Verification items for the finished model (mm, model axes). Round coordinates to 2 decimals unless told otherwise and drop trailing zeros. Order: outer loops, then holes, each group sorted by start corner. A loop starts at its lowest first (then second) coordinate and runs counter-clockwise, first axis right, second up. Notation, with made-up numbers: M 46,17.25 L 53,17.25 A23 cw 53,42.25 Z; hole C 68,1.25 d1. An arc over 180 degrees is marked long. Use CSV: the item, a comma, the result in double quotes. Start each with the question number.
Q1. Sectioned sample at A-A (y = 61.5). Enter the section's corners in (x, z).
Q2. Scan lines: line 1 (X direction, y = 17.5, z = 0.9); line 2 (X direction, y = 81, z = 1.25); line 3 (Z direction, x = -1, y = 69). Record each from-to range of solid material in increasing order.
Q3. Sectioned sample at C-C (z = 3.8). Enter the section's corners in (x, y) (3 decimals), and give its area (3 significant figures).
Q4. Sectioned sample at B-B (x = -1.5). Enter the section's corners in (y, z).
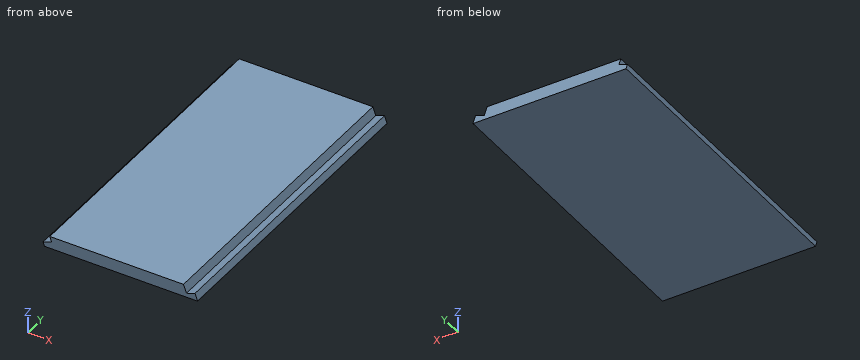
```python
from build123d import *

# Parameters (mm, degrees)
BOX018_W               = 15
BOX018_H               = 100
BOX018_DEPTH           = 3
BOX017_W               = 15
BOX017_H               = 100
BOX017_DEPTH           = 3
BOX016_W               = 27
BOX016_H               = 100
BOX016_DEPTH           = 3
BOX015_W               = 27
BOX015_H               = 100
BOX015_DEPTH           = 3
BOX014_W               = 4
BOX014_H               = 100
BOX014_DEPTH           = 51
BOX014_PITCH_ANGLE     = 20
CUT012_PLACEMENT_ANGLE = 110


with BuildPart() as ranura_superior:
    # Box018 → Box018 (new body)
    with BuildSketch(Plane(origin=(16, 0, 44), x_dir=(1, 0, 0), z_dir=(0, 0, 1))):
        with Locations((7.5, 50)):
            Rectangle(BOX018_W, BOX018_H)
    extrude(amount=BOX018_DEPTH)


with BuildPart() as obj1:
    # Box017 → Box017 (new body)
    with BuildSketch(Plane.XY):
        with Locations((7.5, 50)):
            Rectangle(BOX017_W, BOX017_H)
    extrude(amount=BOX017_DEPTH)


with BuildPart() as obj2:
    # Box016 → Box016 (new body)
    with BuildSketch(Plane(origin=(5, 0, 47), x_dir=(1, 0, 0), z_dir=(0, 0, 1))):
        with Locations((13.5, 50)):
            Rectangle(BOX016_W, BOX016_H)
    extrude(amount=BOX016_DEPTH)


with BuildPart() as obj3:
    # Box015 → Box015 (new body)
    with BuildSketch(Plane(origin=(-9, 0, -3), x_dir=(1, 0, 0), z_dir=(0, 0, 1))):
        with Locations((13.5, 50)):
            Rectangle(BOX015_W, BOX015_H)
    extrude(amount=BOX015_DEPTH)


with BuildPart() as obj4:
    # Box014 → Box014 (new body)
    with BuildSketch(Plane.XY):
        with Locations((2, 50)):
            Rectangle(BOX014_W, BOX014_H)
    extrude(amount=BOX014_DEPTH)


with BuildPart() as obj4_1:
    # Box014 pitch: moved
    add(obj4.part.rotate(Axis((0, 0, 0), (0, 1, 0)), BOX014_PITCH_ANGLE))


with BuildPart() as obj4_2:
    # Box014 placement: moved
    add(obj4_1.part.moved(Location((-2.499695, 0, 0.034905))))

    # Cut009: cut obj3
    add(obj3.part, mode=Mode.SUBTRACT)

    # Cut010: cut obj2
    add(obj2.part, mode=Mode.SUBTRACT)

    # Cut011: cut obj1
    add(obj1.part, mode=Mode.SUBTRACT)

    # Cut012: cut ranura superior
    add(ranura_superior.part, mode=Mode.SUBTRACT)


with BuildPart() as obj4_3:
    # Cut012 placement: moved
    add(obj4_2.part.moved(Location((0, 0, 3))).rotate(Axis((0, 0, 3), (0, -1, 0)), CUT012_PLACEMENT_ANGLE))


solid = obj4_3.part
```
Verdict:
1,outline,"M -49.64,1.96 L -49.16,0.64 L 0.82,0.64 L 0.82,0.74 L 0,3 L -2.82,1.97 L -3.79,4.64 L -47.42,4.64 L -46.82,2.99 Z"
2,line 1,"x = -49.25 to 0.76"
2,line 2,"x = -49.38 to 0.64"
2,line 3,"z = 0.64 to 2.64"
3,outline,"M -47.115,0 L -3.484,0 L -3.484,100 L -47.115,100 Z"
3,area,"4,360 mm²"
4,outline,"M 0,0.64 L 100,0.64 L 100,2.45 L 0,2.45 Z"
